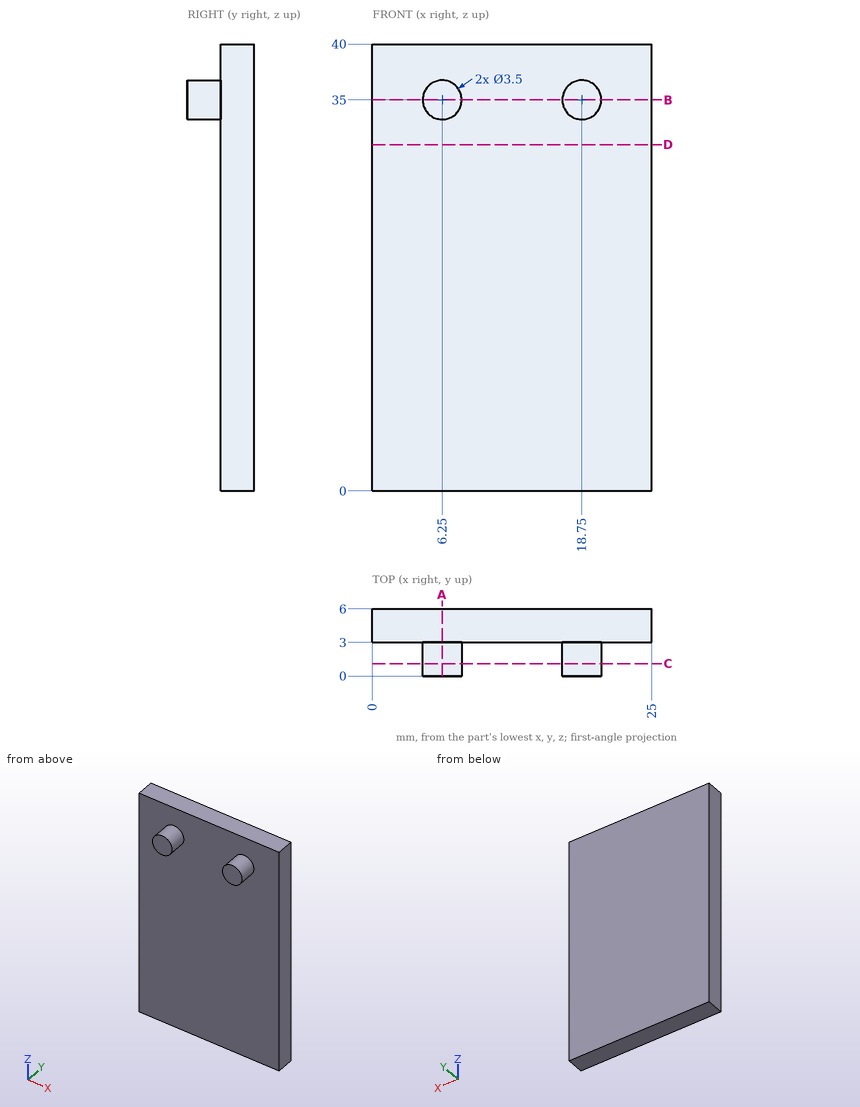
For this review, use the dimensioned drawing (mm, ordinates from the lowest corner) and the shaded views. Round coordinates to 2 decimals unless told otherwise and drop trailing zeros. Order: outer loops, then holes, each group sorted by start corner. A loop starts at its lowest first (then second) coordinate and runs counter-clockwise, first axis right, second up. Notation, with made-up numbers: (20, -37.5) -> (54, -37.5) arc R35 cw to (54, -3.5) -> close; hole circle Ø4 at (61.25, 63). An arc over 180 degrees is marked (long way). Use CSV: the item, a comma, the result in double quotes. Start each with the question number.
(1) Consider section B-B on z = 35. Write out the cut boundary in (x, y).
(2) Consider section C-C on y = 1.1. Write out the cut boundary in (x, z), and give its area (3 significant figures).
(3) Wall thickness on probe 1 along Y at (x, z) = (9.5, 18.5); probe 2 along X at (y, z) = (2.7, 34); probe 3 along Z at (x, y) = (6, 0.85): over which ranges is each line inside the solid? List them lowest first. Write a range as from..to.
(4) Consider section D-D on z = 31. Write out the cut boundary in (x, y).
(5) Consider section A-A on x = 6.25. Write out the cut boundary in (y, z), and give its area (4 significant figures).
Responses:
1,outline,"(0, 3) -> (4.5, 3) -> (4.5, 0) -> (8, 0) -> (8, 3) -> (17, 3) -> (17, 0) -> (20.5, 0) -> (20.5, 3) -> (25, 3) -> (25, 6) -> (0, 6) -> close"
2,outline,"circle Ø3.5 at (6.25, 35); circle Ø3.5 at (18.75, 35)"
2,area,"19.2 mm²"
3,probe 1,"3..6"
3,probe 2,"4.81..7.69, 17.31..20.19"
3,probe 3,"33.27..36.73"
4,outline,"(0, 3) -> (25, 3) -> (25, 6) -> (0, 6) -> close"
5,outline,"(0, 33.25) -> (3, 33.25) -> (3, 0) -> (6, 0) -> (6, 40) -> (3, 40) -> (3, 36.75) -> (0, 36.75) -> close"
5,area,"130.5 mm²"
